Source: three-view drawing plus pictorial views. Frame: mm from the lowest corner of the part. A direction names the side the tool comes from. Give positions to 0.01 mm unless a question says otherwise; leave off trailing zeros. Loops run counter-clockwise (first coordinate to the right, second up) from the corner with the lowest first, then second, coordinate; pieces in that order, holes last. Notation, with made-up numbers: (-22, 84) - (22, 84) arc R27 cw to (22, 106) - close; hole circle Ø2 at (18, 72). An arc over 180 degrees is marked (long way). Answer as a JSON object with one key per item and string values. Group by question number.
(1) Section query D-D (x = 11). Return loops of the section in (y, z) (3 decimals), plus the area to 3 significant figures.
(2) Section query B-B (x = 25.4). Return loops of the section in (y, z) (3 decimals), plus the area to 3 significant figures.
(3) Mould query, pull axis X, two halves, no side actions, for the marked faces 3, 4 and 5. Classes: +X half, -X half, draft (parallel to the pull), parting line (faces both ways), or undercut.
(4) Pin query (flat end, axial travel): P1, Ø10, axis at x = 22, y = 36, coming from the -Z side (3 decimals). Return the tip coordinate at first contact, or that it passes through.
(5) Access query for the marked faces 1 and 2. Directions: +Z, -Z, +X, -X, +Y, -Y. A direction counts if a zero-diameter tool reaches every point of the face in a straight line with its end or side. Return the directions, or none.
(6) Section query C-C (y = 39). Return loops of the section in (x, z) (3 decimals), plus the area to 3 significant figures.
(7) Section query A-A (z = 12). Return loops of the section in (x, y) (3 decimals).
(8) Material intervals for L1, parallel to X at y = 27, z = 17 (3 decimals); L2, parallel to Y at x = 25.4, z = 23.7; L3, parallel to Z at x = 41.5, y = 17.5 (3 decimals), sorted ascending.
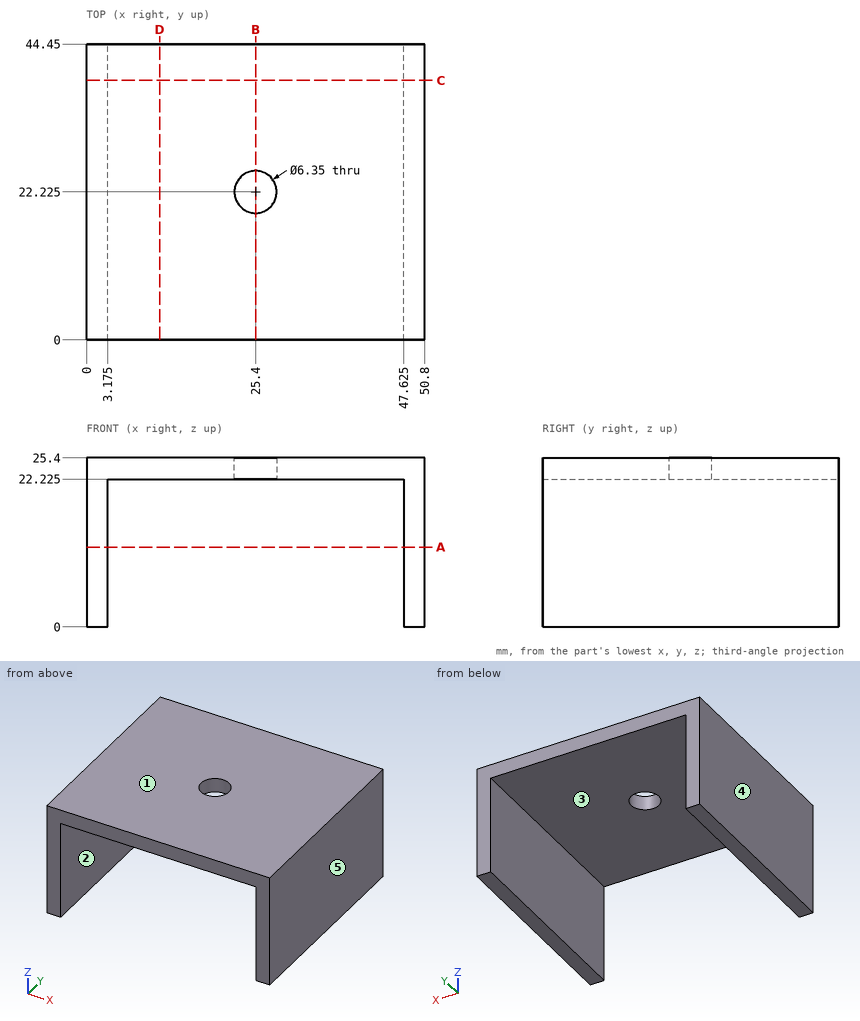
Recorded:
{
 "1": {"outline": "(0, 22.225) - (44.45, 22.225) - (44.45, 25.4) - (0, 25.4) - close", "area": "141 mm^2"},
 "2": {"outline": "(0, 22.225) - (19.05, 22.225) - (19.05, 25.4) - (0, 25.4) - close; (25.4, 22.225) - (44.45, 22.225) - (44.45, 25.4) - (25.4, 25.4) - close", "area": "121 mm^2"},
 "3": {"face 3": "undercut", "face 4": "-X half", "face 5": "+X half"},
 "4": {"P1": "stops at z = 22.225"},
 "5": {"face 1": "+Z, +X, -X, +Y, -Y", "face 2": "-Z, +Y, -Y"},
 "6": {"outline": "(0, 0) - (3.175, 0) - (3.175, 22.225) - (47.625, 22.225) - (47.625, 0) - (50.8, 0) - (50.8, 25.4) - (0, 25.4) - close", "area": "302 mm^2"},
 "7": {"outline": "(0, 0) - (3.175, 0) - (3.175, 44.45) - (0, 44.45) - close; (47.625, 0) - (50.8, 0) - (50.8, 44.45) - (47.625, 44.45) - close"},
 "8": {"L1": "x = 0 to 3.175, 47.625 to 50.8", "L2": "y = 0 to 19.05, 25.4 to 44.45", "L3": "z = 22.225 to 25.4"}
}
